Geometry: final body of the model. Coordinates: model frame, mm. Give positions to 0.01 mm unless a question says otherwise; leave off trailing zeros. Write each loop counter-clockwise with the first axis right and the second up, starting at its lowest first coordinate (ties: lowest second). Pieces come first, ordered by that corner, then holes. Notation, with made-up numbers: (43, 19) -> (79, 19) arc R16 ccw to (79, 30) -> close; hole circle Ø3 at (56, 71). An arc over 180 degrees is marked (long way). Answer as a JSON object with one key per item and string values.
from build123d import *

# Parameters (mm, degrees)
F1_DEPTH       = 9.525
F2_D           = 5.5
F2_CBORE_D     = 9.75
F2_CBORE_DEPTH = 5
F3_R           = 5.08
F4_DEPTH       = 5
F5_D           = 5.5


# Not quite as in the source:
# - a feature names something its author has since deleted; it is built from what else it names


with BuildPart() as f1:
    # F0 (on Front) → F1 (new body)
    with BuildSketch(Plane.XZ):
        with BuildLine():
            Line((10, -40), (10, 0))
            ThreePointArc((10, 0), (7.0710678119, 7.0710678119), (0, 10))
            Line((0, 10), (-53.34, 10))
            ThreePointArc((-53.34, 10), (-62.826927837, 3.1619930765), (-59.3395200276, -8.0003599568))
            Line((-59.3395200276, -8.0003599568), (-5.9995200276, -48.0003599568))
            ThreePointArc((-5.9995200276, -48.0003599568), (4.4724042597, -48.9441377526), (10, -40))
        make_face()
        Polygon((-17.9525227119, 0), (-20.4062613559, -4.25), (-25.3137386441, -4.25), (-27.7674772881, 0), (-25.3137386441, 4.25), (-20.4062613559, 4.25), align=None, mode=Mode.SUBTRACT)
        Polygon((-25.3137386441, -4.25), (-20.4062613559, -4.25), (-17.9525227119, 0), (-20.4062613559, 4.25), (-25.3137386441, 4.25), (-27.7674772881, 0), align=None)
    extrude(amount=-F1_DEPTH)

    # F2 (through all)
    with Locations(Plane.XZ):
        with Locations((0, 0), (0, -40), (-53.34, 0)):
            CounterBoreHole(F2_D / 2, F2_CBORE_D / 2, F2_CBORE_DEPTH)

    # F3
    f3_edges = [f1.edges().sort_by_distance(p)[0] for p in [
        (-26.67, 0, 10),
    ]]
    fillet(f3_edges, radius=F3_R)

    # F0 (on Front) → F4 (cut)
    with BuildSketch(Plane.XZ):
        Polygon((-25.3137386441, -4.25), (-20.4062613559, -4.25), (-17.9525227119, 0), (-20.4062613559, 4.25), (-25.3137386441, 4.25), (-27.7674772881, 0), align=None)
    extrude(amount=-F4_DEPTH, mode=Mode.SUBTRACT)

    # F5 (through all)
    with Locations(Plane.XZ):
        with Locations((-22.86, 0)):
            Hole(F5_D / 2)


solid = f1.part
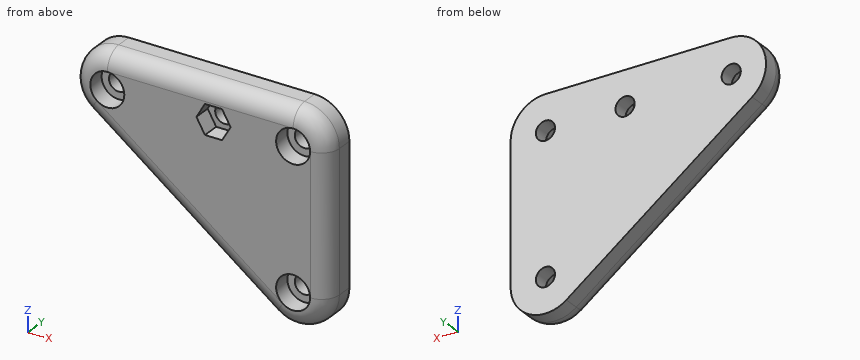
Q1. First-contact query: P1, Ø6.5, axis at x = -22.86, z = 0, coming from the -Y side; P2, Ø5.5, axis at x = -22.5, y = 1.5, coming from the +Z side; P3, Ø12, axis at x = -15.5, z = -41, coming from the +Y side (3 decimals); P4, Ø2, axis at x = -8, y = 5, coming from the -Z side. Flat tips, straight axial feed; report the tip coordinate or a pass-through.
Values:
{"P1": "y = 5", "P2": "z = 9.93", "P3": "y = 9.525", "P4": "z = -47.25"}
Q2. Material intervals for L1, parallel to Z at x = 0, y = 8.4; L2, parallel to Z at x = 4, y = 3; L3, parallel to X at y = 2.75, z = -42, sorted ascending. Write a range as from..to.
Values:
{"L1": "-50..-42.75, -37.25..-2.75, 2.75..10", "L2": "-48.68..-42.79, -37.21..-2.79, 2.79..8.68", "L3": "-13.06..-4.45, 4.45..9.22"}
Q3. Cut plane A-A (y = 8.5). Return the cut outline in (x, z).
Values:
{"outline": "(-59.34, -8) -> (-6, -48) arc R10 ccw to (10, -40) -> (10, 0) arc R10 ccw to (0, 10) -> (-53.34, 10) arc R10 ccw to start; hole circle Ø5.5 at (-53.34, 0); hole circle Ø5.5 at (-22.86, 0); hole circle Ø5.5 at (0, -40); hole circle Ø5.5 at (0, 0)"}
Q4. Cut plane B-B (z = 1.5). State how many separate pieces and enclosed holes the cut face has, and give its area (3 significant figures).
Values:
{"separate pieces": "4", "enclosed holes": "0", "area": "489 mm²"}
